Verification items for the finished model (mm, model axes). Coordinates: 2 decimals unless noted, no trailing zeros. Write each loop counter-clockwise with the first axis right and the second up, starting at its lowest first coordinate (ties: lowest second). Pieces come first, ordered by that corner, then holes. Notation, with made-up numbers: (41, 25.25) -> (73, 25.25) arc R27 ccw to (73, 41.25) -> close; hole circle Ø5 at (40.5, 25). An arc over 180 degrees is marked (long way). Answer in a Markdown table with one row per item.
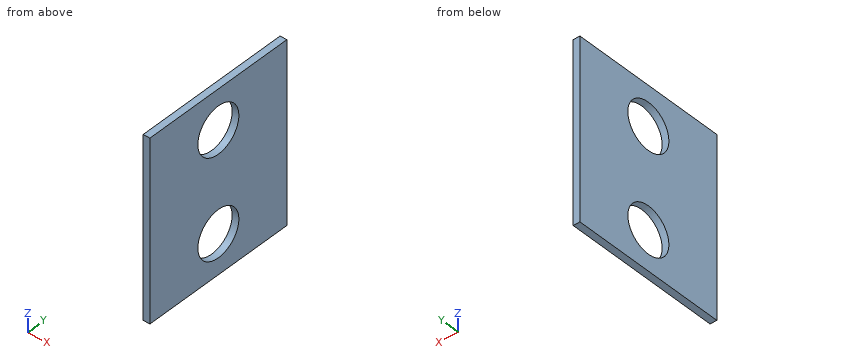
```python
from build123d import *

# Parameters (mm, degrees)
FLANGE_BASE1_START     = -0.5
FLANGE_BASE1_OUTLINE_W = 26.9
FLANGE_BASE1_OUTLINE_H = 23.35
FLANGE_BASE1_DEPTH     = 1
ESBO_O2_R              = 3.5
CORTE_EXTRUS_O1_DEPTH  = 1


# Read off the part's stored shape, not the designer's step: Flange-base1
with BuildPart() as part:
    # Flange-base1 outline → Flange-base1 (new body)
    with BuildSketch(Plane(origin=(0, 0, 0), x_dir=(0, 0, -1), z_dir=(1, 0, 0)).offset(FLANGE_BASE1_START)):
        Rectangle(FLANGE_BASE1_OUTLINE_W, FLANGE_BASE1_OUTLINE_H)
    extrude(amount=FLANGE_BASE1_DEPTH)

    # Esboço2 → Corte-extrusão1 (cut)
    with BuildSketch(Plane.ZY.offset(0.5)):
        with Locations((-7.5, 0)):
            Circle(ESBO_O2_R)
        with Locations((7.5, 0)):
            Circle(ESBO_O2_R)
    extrude(amount=-CORTE_EXTRUS_O1_DEPTH, mode=Mode.SUBTRACT)


solid = part.part
```
1. Sectioned sample at A-A, the plane z = 7.5. Record the cut outline in (x, y) (3 decimals), and give its area (4 significant figures).
Findings below:
| item | result |
|---|---|
| outline | (-0.5, -11.675) -> (0.5, -11.675) -> (0.5, -3.5) -> (-0.5, -3.5) -> close; (-0.5, 3.5) -> (0.5, 3.5) -> (0.5, 11.675) -> (-0.5, 11.675) -> close |
| area | 16.35 mm² |
2. Sectioned sample at C-C, the plane x = -0.1. Record the cut outline in (y, z) (3 decimals), and give its area (3 significant figures).
Findings below:
| item | result |
|---|---|
| outline | (-11.675, -13.45) -> (11.675, -13.45) -> (11.675, 13.45) -> (-11.675, 13.45) -> close; hole circle Ø7 at (0, -7.5); hole circle Ø7 at (0, 7.5) |
| area | 551 mm² |
3. Sectioned sample at D-D, the plane z = -6. Record the cut outline in (x, y) (3 decimals), and give its area (3 significant figures).
Findings below:
| item | result |
|---|---|
| outline | (-0.5, -11.675) -> (0.5, -11.675) -> (0.5, -3.162) -> (-0.5, -3.162) -> close; (-0.5, 3.162) -> (0.5, 3.162) -> (0.5, 11.675) -> (-0.5, 11.675) -> close |
| area | 17.0 mm² |
4. Material ranges on probe 1 along Y at (x, z) = (-0.1, 7.5) (3 decimals); probe 2 along Z at (x, y) = (-0.4, -0.75); probe 3 along Z at (x, y) = (-0.2, -1.5), recorded low to high. Write a range as from..to.
Findings below:
| item | result |
|---|---|
| probe 1 | y = -11.675..-3.5, 3.5..11.675 |
| probe 2 | z = -13.45..-10.92, -4.08..4.08, 10.92..13.45 |
| probe 3 | z = -13.45..-10.66, -4.34..4.34, 10.66..13.45 |
5. Go/stop test with a flat-tipped pin: pin 1 (4 mm diameter, centred on y = 0, z = 7.5, fed in from +X). Record where the tip stops, or that it passes through.
Findings below:
| item | result |
|---|---|
| pin 1 | passes through |
6. Sectioned sample at B-B, the plane y = 0. Record the cut outline in (x, z), and give its area (3 significant figures).
Findings below:
| item | result |
|---|---|
| outline | (-0.5, -13.45) -> (0.5, -13.45) -> (0.5, -11) -> (-0.5, -11) -> close; (-0.5, -4) -> (0.5, -4) -> (0.5, 4) -> (-0.5, 4) -> close; (-0.5, 11) -> (0.5, 11) -> (0.5, 13.45) -> (-0.5, 13.45) -> close |
| area | 12.9 mm² |
